Source: three-view drawing plus pictorial views. Frame: mm from the lowest corner of the part. Give positions to 0.01 mm unless a question says otherwise; leave off trailing zeros. Order: outer loops, then holes, each group sorted by start corner. A loop starts at its lowest first (then second) coordinate and runs counter-clockwise, first axis right, second up.
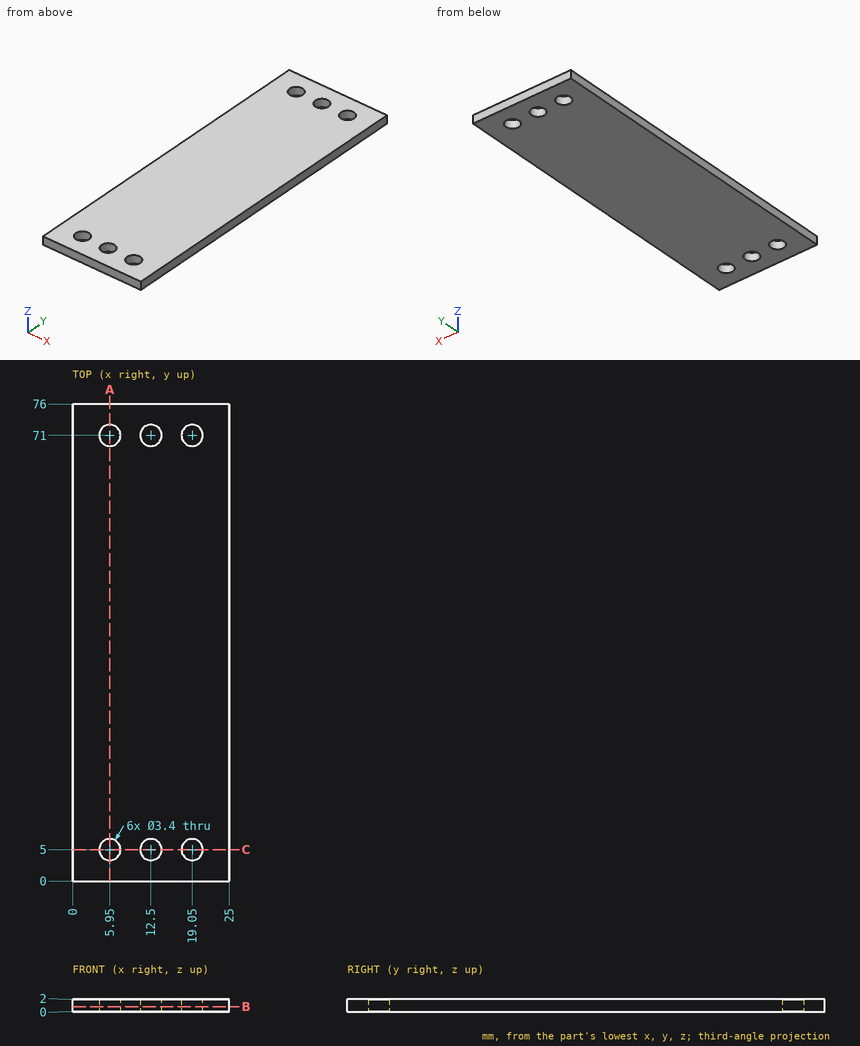
1) Section query C-C on y = 5. Output: boundary loops of the cut face in (x, z), and give its area (3 significant figures).
Checks:
outline: (0, 0) - (4.25, 0) - (4.25, 2) - (0, 2) - close; (7.65, 0) - (10.8, 0) - (10.8, 2) - (7.65, 2) - close; (14.2, 0) - (17.35, 0) - (17.35, 2) - (14.2, 2) - close; (20.75, 0) - (25, 0) - (25, 2) - (20.75, 2) - close
area: 29.6 mm2
2) Section query B-B on z = 0.8. Output: boundary loops of the cut face in (x, y).
Checks:
outline: (0, 0) - (25, 0) - (25, 76) - (0, 76) - close; hole circle Ø3.4 at (5.95, 5); hole circle Ø3.4 at (5.95, 71); hole circle Ø3.4 at (12.5, 5); hole circle Ø3.4 at (12.5, 71); hole circle Ø3.4 at (19.05, 5); hole circle Ø3.4 at (19.05, 71)
3) Ray query, L1, parallel to Y at x = 5.95, z = 0.6; L2, parallel to X at y = 71, z = 0.7; L3, parallel to X at y = 70, z = 1.7. Return the intervals inside material, ascending.
Checks:
L1: y = 0 to 3.3, 6.7 to 69.3, 72.7 to 76
L2: x = 0 to 4.25, 7.65 to 10.8, 14.2 to 17.35, 20.75 to 25
L3: x = 0 to 4.58, 7.32 to 11.13, 13.87 to 17.68, 20.42 to 25
4) Section query A-A on x = 5.95. Output: boundary loops of the cut face in (y, z), and give its area (3 significant figures).
Checks:
outline: (0, 0) - (3.3, 0) - (3.3, 2) - (0, 2) - close; (6.7, 0) - (69.3, 0) - (69.3, 2) - (6.7, 2) - close; (72.7, 0) - (76, 0) - (76, 2) - (72.7, 2) - close
area: 138 mm2
